Autodesk Inventor part; units mm, degrees
ref_plane "YZ Plane" through (0, 0, 0) normal (1, 0, 0) x (0, 1, 0)
ref_plane "XZ Plane" through (0, 0, 0) normal (0, 1, 0) x (-1, 0, 0)
ref_plane "XY Plane" through (0, 0, 0) normal (0, 0, 1) x (1, 0, 0)
sketch "Sketch1" plane through (0, 0, 0) normal (0, 0, 1) x (1, 0, 0)
  circle A0 centre (0, 0) radius 52.5 construction
  circle A1 centre (0, 0) radius 25
  circle A2 centre (0, 0) radius 62.5
  line L0 (0, 0) -> (0, 52.5) construction
  line L1 (0, 0) -> (37.1231, 37.1231) construction
  line L2 (0, 0) -> (0, -125) construction
  circle A3 centre (0, -125) radius 87.5
  line L3 (-85.7321, -107.5) -> (-61.2372, 12.5)
  line L4 (85.7321, -107.5) -> (61.2372, 12.5)
  circle A4 centre (0, -125) radius 25
  circle A5 centre (0, -125) radius 81 construction
  circle A6 centre (0, 0) radius 56 construction
  line L5 (0, 0) -> (-56, 0) construction
  line L6 (0, -125) -> (-81, -125) construction
  dimension "d31" = 162
  dimension "d32" = 112
  dimension "d0" = 105
  dimension "d1" = 50
  dimension "d2" = 125
  dimension "d3" = 45
  dimension "d4" = 125
  dimension "d5" = 175
  dimension "d6" = 50
extrude "Extrusion1" add sketch "Sketch1" along normal blind 3
sketch "Sketch2" plane through (0, 0, 0) normal (0, 0, 1) x (1, 0, 0)
  line L0 (0, 0) -> (0, -100)
  line L1 (67.5, -100) -> (-67.5, -100)
  arc A0 (-85.7321, -107.5) -> (85.7321, -107.5) centre (0, -125) ccw
  dimension "d11" = 100
  dimension "d12" = 135
  dimension "d40" = 25
hole "Hole1" at (67.5, -100, 0) at (-67.5, -100, 0) direction (0, 0, 1) diameter 6.6 end through all
hole "Hole2" at (37.1231, 37.1231, 0) direction (0, 0, 1) diameter 5.5 end through all
pattern_circular "Circular Pattern1" count 4 over 360 about axis through (0, 0, 0) along (0, 0, 1) of "Hole2"
hole "Hole3" at (-56, 0, 0) at (-81, -125, 0) direction (0, 0, 1) diameter 9 end through all
mirror "Mirror1" about plane through (0, 0, 0) normal (1, 0, 0) of "Hole3"
properties part number "PWTR-0128" material "Aluminum 6061"
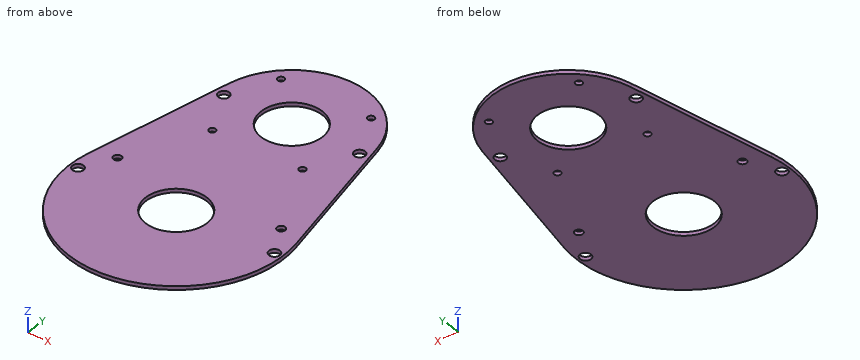
The listing builds one solid part. Answer for the finished solid, in the listing's coordinates (mm). Coordinates: 2 decimals unless noted, no trailing zeros. Write each loop counter-clockwise with the first axis right and the second up, starting at its lowest first coordinate (ties: lowest second). Pieces come first, ordered by that corner, then holes. Notation, with made-up numbers: (-39.5, 66) - (-17.5, 66) arc R30 ccw to (-17.5, 100) - close; hole circle Ø10 at (-30, -21). An arc over 180 degrees is marked (long way). Return JSON: item names as keys, results as strings. Group by question number.
Q1. Flat-ended cylindrical pins translate along their axes: pin 1 Ø7 at (x, y) = (37.12, -37.12) entering from +Z; pin 2 Ø1 at (y, z) = (-113.5, 2.5) entering from -X. Find the tip coordinate at first contact, or state that the pin passes through.
Q2. The part is cut by section A-A on y = -125. Write down the section's boundary in (x, z).
Q3. The part is cut by section C-C on z = 1.35. State how many separate pieces and enclosed holes the cut face has, and give its area (3 significant figures).
Q4. Find the intervals of material crossed by line 1 along Y through (x, z) = (-14.5, 2.45); line 2 along Y through (x, z) = (-22.5, 1.5); line 3 along X through (y, z) = (-35, 1.65), in increasing order. Write a range as [from, to].
Q5. The part is cut by section D-D on x = -19. Write down the section's boundary in (y, z).
Q6. The part is cut by section B-B on x = 67.5. Write down the section's boundary in (y, z).
Evaluation:
{
 "1": {"pin 1": "stops at z = 3", "pin 2": "stops at x = -86.81"},
 "2": {"outline": "(-87.5, 0) - (-85.5, 0) - (-85.5, 3) - (-87.5, 3) - close; (-76.5, 0) - (-25, 0) - (-25, 3) - (-76.5, 3) - close; (25, 0) - (76.5, 0) - (76.5, 3) - (25, 3) - close; (85.5, 0) - (87.5, 0) - (87.5, 3) - (85.5, 3) - close"},
 "3": {"separate pieces": "1", "enclosed holes": "12", "area": "32,900 mm2"},
 "4": {"line 1": "y = [-211.29, -145.37], [-104.63, -20.37], [20.37, 60.79]", "line 2": "y = [-209.56, -135.9], [-114.1, -10.9], [10.9, 58.31]", "line 3": "x = [-70.93, -38.87], [-35.38, 35.38], [38.87, 70.93]"},
 "5": {"outline": "(-210.41, 0) - (-141.25, 0) - (-141.25, 3) - (-210.41, 3) - close; (-108.75, 0) - (-16.25, 0) - (-16.25, 3) - (-108.75, 3) - close; (16.25, 0) - (59.54, 0) - (59.54, 3) - (16.25, 3) - close"},
 "6": {"outline": "(-180.68, 0) - (-103.3, 0) - (-103.3, 3) - (-180.68, 3) - close; (-96.7, 0) - (-18.18, 0) - (-18.18, 3) - (-96.7, 3) - close"}
}
